CAD build for the part. Positions are in the model's coordinates, mm. A direction names the side the tool comes from. Round coordinates to 2 decimals unless told otherwise and drop trailing zeros. Order: outer loops, then holes, each group sorted by start corner. A loop starts at its lowest first (then second) coordinate and runs counter-clockwise, first axis right, second up. Notation, with made-up numbers: (48.25, 79.5) - (67.25, 79.5) arc R18 ccw to (67.25, 99.5) - close; hole circle Ø6 at (11, 78). An arc over 180 degrees is marked (long way). Write item = value, one per line.
from build123d import *

# Parameters (mm, degrees)
SKETCH1_W           = 130
SKETCH1_H           = 45
BOSS_EXTRUDE1_DEPTH = 42
SKETCH2_W           = 10
SKETCH2_H           = 22
CUT_EXTRUDE1_DEPTH  = 115
SKETCH3_W           = 41
SKETCH3_H           = 41
CUT_EXTRUDE2_DEPTH  = 12
CUT_EXTRUDE3_START  = -26.05
SKETCH5_W           = 49
SKETCH5_H           = 45
CUT_EXTRUDE3_DEPTH  = 26.05
SKETCH6_R           = 2
CUT_EXTRUDE4_DEPTH  = 43
SKETCH7_R           = 12
CUT_EXTRUDE5_DEPTH  = 3.5
SKETCH8_R           = 7.5
CUT_EXTRUDE6_DEPTH  = 46
SKETCH10_W          = 23
SKETCH10_H          = 28
CUT_EXTRUDE7_DEPTH  = 46
FILLET1_R           = 5
SKETCH11_R          = 5.75
CUT_EXTRUDE8_DEPTH  = 42.5
SKETCH12_R          = 1.35
CUT_EXTRUDE9_DEPTH  = 20
SKETCH14_R          = 1.75
CUT_EXTRUDE11_DEPTH = 12
SKETCH15_W          = 32.462008986
SKETCH15_H          = 10
CUT_EXTRUDE12_DEPTH = 46
FILLET2_R           = 5
FILLET3_R           = 5
SKETCH16_R          = 12.5
CUT_EXTRUDE13_DEPTH = 33.5
SKETCH17_W          = 2.5
SKETCH17_H          = 24
BOSS_EXTRUDE2_DEPTH = 10
SKETCH18_R          = 1.35
CUT_EXTRUDE14_DEPTH = 10
FILLET4_R           = 3
FILLET5_R           = 3
SKETCH20_W          = 5
SKETCH20_H          = 1.4
BOSS_EXTRUDE3_DEPTH = 2.8
SKETCH22_W          = 5
SKETCH22_H          = 1.4
BOSS_EXTRUDE4_DEPTH = 2.8
SKETCH25_W          = 1.5
SKETCH25_H          = 5
SKETCH25_W_2        = 5
SKETCH25_H_2        = 1.5
BOSS_EXTRUDE5_DEPTH = 7
SKETCH26_R          = 14.5
CUT_EXTRUDE15_DEPTH = 10
SKETCH27_W          = 6
SKETCH27_H          = 11
CUT_EXTRUDE16_DEPTH = 10


with BuildPart() as part:
    # Sketch1 → Boss-Extrude1 (new body)
    with BuildSketch(Plane.XY):
        with Locations((65, 22.5)):
            Rectangle(SKETCH1_W, SKETCH1_H)
    extrude(amount=BOSS_EXTRUDE1_DEPTH)

    # Sketch2 → Cut-Extrude1 (cut)
    with BuildSketch(Plane.ZY):
        with Locations((7, 22.5)):
            Rectangle(SKETCH2_W, SKETCH2_H)
    extrude(amount=-CUT_EXTRUDE1_DEPTH, mode=Mode.SUBTRACT)

    # Sketch3 → Cut-Extrude2 (cut)
    with BuildSketch(Plane(origin=(0, 0, 0), x_dir=(-1, 0, 0), z_dir=(0, 0, -1))):
        with Locations((-103, 22.5)):
            Rectangle(SKETCH3_W, SKETCH3_H)
    extrude(amount=-CUT_EXTRUDE2_DEPTH, mode=Mode.SUBTRACT)

    # Sketch5 → Cut-Extrude3 (cut)
    with BuildSketch(Plane.XY.offset(42).offset(CUT_EXTRUDE3_START)):
        with Locations((105.5, 22.5)):
            Rectangle(SKETCH5_W, SKETCH5_H)
    extrude(amount=CUT_EXTRUDE3_DEPTH, mode=Mode.SUBTRACT)

    # Sketch6 → Cut-Extrude4 (cut, through all)
    with BuildSketch(Plane(origin=(0, 0, 0), x_dir=(-1, 0, 0), z_dir=(0, 0, -1))):
        with Locations((-118.5, 38)):
            Circle(SKETCH6_R)
        with Locations((-87.5, 38)):
            Circle(SKETCH6_R)
        with Locations((-87.5, 7)):
            Circle(SKETCH6_R)
        with Locations((-118.5, 7)):
            Circle(SKETCH6_R)
    extrude(amount=-CUT_EXTRUDE4_DEPTH, mode=Mode.SUBTRACT)

    # Sketch7 → Cut-Extrude5 (cut)
    with BuildSketch(Plane(origin=(0, 45, 0), x_dir=(1, 0, 0), z_dir=(0, 1, 0))):
        with Locations((38.5, -21)):
            Circle(SKETCH7_R)
    extrude(amount=-CUT_EXTRUDE5_DEPTH, mode=Mode.SUBTRACT)

    # Sketch8 → Cut-Extrude6 (cut, through all)
    with BuildSketch(Plane(origin=(0, 45, 0), x_dir=(1, 0, 0), z_dir=(0, 1, 0))):
        with Locations((68.5, -21)):
            Circle(SKETCH8_R)
    extrude(amount=-CUT_EXTRUDE6_DEPTH, mode=Mode.SUBTRACT)

    # Sketch10 → Cut-Extrude7 (cut, through all)
    with BuildSketch(Plane(origin=(0, 45, 0), x_dir=(1, 0, 0), z_dir=(0, 1, 0))):
        with Locations((11.5, -28)):
            Rectangle(SKETCH10_W, SKETCH10_H)
    extrude(amount=-CUT_EXTRUDE7_DEPTH, mode=Mode.SUBTRACT)

    # Fillet1
    fillet1_edges = [part.edges().sort_by_distance(p)[0] for p in [
        (23, 22.5, 42),
        (81, 22.5, 42),
    ]]
    fillet(fillet1_edges, radius=FILLET1_R)

    # Sketch11 → Cut-Extrude8 (cut, through all)
    with BuildSketch(Plane(origin=(0, 41.5, 0), x_dir=(1, 0, 0), z_dir=(0, 1, 0))):
        with Locations((38.5, -21)):
            Circle(SKETCH11_R)
    extrude(amount=-CUT_EXTRUDE8_DEPTH, mode=Mode.SUBTRACT)

    # Sketch12 → Cut-Extrude9 (cut)
    with BuildSketch(Plane(origin=(0, 41.5, 0), x_dir=(1, 0, 0), z_dir=(0, 1, 0))):
        with Locations((32.843145751, -15.343145751)):
            Circle(SKETCH12_R)
        with Locations((44.156854249, -15.343145751)):
            Circle(SKETCH12_R)
        with Locations((44.156854249, -26.656854249)):
            Circle(SKETCH12_R)
        with Locations((32.843145751, -26.656854249)):
            Circle(SKETCH12_R)
    extrude(amount=-CUT_EXTRUDE9_DEPTH, mode=Mode.SUBTRACT)

    # Sketch14 → Cut-Extrude11 (cut)
    with BuildSketch(Plane(origin=(0, 0, 0), x_dir=(-1, 0, 0), z_dir=(0, 0, -1))):
        with Locations((-75, 37.5)):
            Circle(SKETCH14_R)
        with Locations((-15, 37.5)):
            Circle(SKETCH14_R)
        with Locations((-15, 7.5)):
            Circle(SKETCH14_R)
        with Locations((-75, 7.5)):
            Circle(SKETCH14_R)
    extrude(amount=-CUT_EXTRUDE11_DEPTH, mode=Mode.SUBTRACT)

    # Sketch15 → Cut-Extrude12 (cut, through all)
    with BuildSketch(Plane(origin=(0, 45, 0), x_dir=(1, 0, 0), z_dir=(0, 1, 0))):
        with Locations((82.343987658, -21)):
            Rectangle(SKETCH15_W, SKETCH15_H)
    extrude(amount=-CUT_EXTRUDE12_DEPTH, mode=Mode.SUBTRACT)

    # Fillet2
    fillet2_edges = [part.edges().sort_by_distance(p)[0] for p in [
        (81, 22.5, 26),
    ]]
    fillet(fillet2_edges, radius=FILLET2_R)

    # Fillet3
    fillet3_edges = [part.edges().sort_by_distance(p)[0] for p in [
        (23, 22.5, 14),
    ]]
    fillet(fillet3_edges, radius=FILLET3_R)

    # Sketch16 → Cut-Extrude13 (cut)
    with BuildSketch(Plane.XZ):
        with Locations((38.5, 21)):
            Circle(SKETCH16_R)
    extrude(amount=-CUT_EXTRUDE13_DEPTH, mode=Mode.SUBTRACT)

    # Sketch17 → Boss-Extrude2 (add)
    with BuildSketch(Plane.XY.offset(14)):
        with Locations((5.25, 27.5)):
            Rectangle(SKETCH17_W, SKETCH17_H)
    extrude(amount=BOSS_EXTRUDE2_DEPTH)

    # Sketch18 → Cut-Extrude14 (cut)
    with BuildSketch(Plane.ZY.offset(-4)):
        with Locations((19, 36.775)):
            Circle(SKETCH18_R)
        with Locations((19, 17.725)):
            Circle(SKETCH18_R)
    extrude(amount=-CUT_EXTRUDE14_DEPTH, mode=Mode.SUBTRACT)

    # Fillet4
    fillet4_edges = [part.edges().sort_by_distance(p)[0] for p in [
        (6.5, 27.5, 14),
    ]]
    fillet(fillet4_edges, radius=FILLET4_R)

    # Fillet5
    fillet5_edges = [part.edges().sort_by_distance(p)[0] for p in [
        (8, 39.5, 14),
        (8, 15.5, 14),
    ]]
    fillet(fillet5_edges, radius=FILLET5_R)

    # Sketch20 → Boss-Extrude3 (add)
    with BuildSketch(Plane.XY.offset(42)):
        with Locations((30.5, 0.7)):
            Rectangle(SKETCH20_W, SKETCH20_H)
        with Locations((73.5, 0.7)):
            Rectangle(SKETCH20_W, SKETCH20_H)
    extrude(amount=BOSS_EXTRUDE3_DEPTH)

    # Sketch22 → Boss-Extrude4 (add)
    with BuildSketch(Plane.ZY.offset(-23)):
        with Locations((28, 0.7)):
            Rectangle(SKETCH22_W, SKETCH22_H)
    extrude(amount=BOSS_EXTRUDE4_DEPTH)

    # Sketch25 → Boss-Extrude5 (add)
    with BuildSketch(Plane(origin=(0, 1.4, 0), x_dir=(1, 0, 0), z_dir=(0, 1, 0))):
        with Locations((20.95, -28)):
            Rectangle(SKETCH25_W, SKETCH25_H)
        with Locations((73.5, -44.05)):
            Rectangle(SKETCH25_W_2, SKETCH25_H_2)
        with Locations((30.5, -44.05)):
            Rectangle(SKETCH25_W_2, SKETCH25_H_2)
    extrude(amount=BOSS_EXTRUDE5_DEPTH)

    # Sketch26 → Cut-Extrude15 (cut)
    with BuildSketch(Plane(origin=(0, 0, 12), x_dir=(-1, 0, 0), z_dir=(0, 0, -1))):
        with Locations((-103, 22.5)):
            Circle(SKETCH26_R)
    extrude(amount=-CUT_EXTRUDE15_DEPTH, mode=Mode.SUBTRACT)

    # Sketch27 → Cut-Extrude16 (cut)
    with BuildSketch(Plane.ZY.offset(-4)):
        with Locations((19, 27.5)):
            Rectangle(SKETCH27_W, SKETCH27_H)
    extrude(amount=-CUT_EXTRUDE16_DEPTH, mode=Mode.SUBTRACT)


solid = part.part
(1) Band-saw the part on A-A on x = 68.5. List the corners of the cut face in (y, z), plus the area to 3 significant figures.
Solved:
outline = (0, 0) - (45, 0) - (45, 13.5) - (0, 13.5) - close; (0, 28.5) - (45, 28.5) - (45, 42) - (0, 42) - close; hole (11.5, 2) - (33.5, 2) - (33.5, 12) - (11.5, 12) - close
area = 995 mm²
(2) Probe line 1 along Y through (x, z) = (5.4, 19) (3 decimals); line 2 along Y through (x, z) = (52, 10.5); line 3 along Y through (x, z) = (75, 4). List the from-to ranges inside material, lowest first.
Solved:
line_1 = 15.5 to 16.375, 19.075 to 22, 33 to 35.425, 38.125 to 39.5
line_2 = 0 to 11.5, 33.5 to 45
line_3 = 0 to 5.75, 9.25 to 11.5, 33.5 to 35.75, 39.25 to 45
(3) Drop flat-ended pins along their axis: pin 1 (4 mm diameter, centred on x = 15, y = 7.5, fed in from -Z); pin 2 (1.4 mm diameter, centred on x = 22, z = 28.5, fed in from +Y); pin 3 (0.8 mm diameter, centred on y = 5, z = 43, fed in from -X); pin 4 (8 mm diameter, centred on x = 64.5, y = 6.5, fed in from +Z). Give the stop position or say it passes through.
Solved:
pin_1 = 0
pin_2 = 8.4
pin_3 = 28
pin_4 = 42
(4) Band-saw the part on D-D on x = 15. List the corners of the cut face in (y, z).
Solved:
outline = (0, 0) - (5.75, 0) - (5.75, 12) - (9.25, 12) - (9.25, 0) - (35.75, 0) - (35.75, 12) - (39.25, 12) - (39.25, 0) - (45, 0) - (45, 14) - (0, 14) - close; hole (11.5, 2) - (33.5, 2) - (33.5, 12) - (11.5, 12) - close
(5) Pull direction X, two halves, no side cores. Call faces 6 (the flat face through (103, 43, 6)), 7 (the flat face through (15, 8, 12)), 8 (the flat face through (4, 27.3, 15.6)), 9 (the flat face through (5, 22, 19)): released by +X, released by -X, zero draft, split by the parting line, or undercut.
Solved:
face_6 = undercut
face_7 = undercut
face_8 = released by -X
face_9 = zero draft
(6) Band-saw the part on B-B on z = 6. List the corners of the cut face in (x, y), plus the area to 3 significant figures.
Solved:
outline = (0, 0) - (130, 0) - (130, 45) - (0, 45) - (0, 33.5) - (82.5, 33.5) - (82.5, 43) - (123.5, 43) - (123.5, 2) - (82.5, 2) - (82.5, 11.5) - (0, 11.5) - close; hole circle Ø3.5 at (15, 7.5); hole circle Ø3.5 at (15, 37.5); hole circle Ø3.5 at (75, 7.5); hole circle Ø3.5 at (75, 37.5)
area = 2,320 mm²
(7) Tool access for faces 1 (the cylindrical face through (36.873, 16.516, 33.394)), 2 (the flat face through (5, 39.5, 20)), 3 (the flat face through (71, 3, 44)), 4 (the flat face through (77, 23, 16)), 5 (the flat face through (123.5, 22, 6)): list every direction of +Z, -Z, +X, -X, +Y, -Y with a clear straight run to the whole face (end or side of a thin tool).
Solved:
face_1 = -Y
face_2 = +Z, -X, +Y
face_3 = +Z, +Y, -Y
face_4 = +X, +Y, -Y
face_5 = -Z
(8) Band-saw the part on C-C on x = 38.5. List the corners of the cut face in (y, z), plus the area to 4 significant figures.
Solved:
outline = (0, 0) - (45, 0) - (45, 9) - (41.5, 9) - (41.5, 15.25) - (33.5, 15.25) - (33.5, 2) - (11.5, 2) - (11.5, 8.5) - (0, 8.5) - close; (0, 33.5) - (33.5, 33.5) - (33.5, 26.75) - (41.5, 26.75) - (41.5, 33) - (45, 33) - (45, 42) - (0, 42) - close
area = 733.5 mm²
